```python
from build123d import *

# Parameters (mm, degrees)
SKETCH1_W           = 25
SKETCH1_H           = 15
BOSS_EXTRUDE1_DEPTH = 5
SKETCH2_R           = 1
SKETCH2_R_2         = 0.75
BOSS_EXTRUDE2_DEPTH = 5
SKETCH3_R           = 0.75
BOSS_EXTRUDE3_DEPTH = 5


with BuildPart() as part:
    # Sketch1 → Boss-Extrude1 (new body)
    with BuildSketch(Plane(origin=(0, 0, 0), x_dir=(1, 0, 0), z_dir=(0, 1, 0))):
        with Locations((12.5, 7.5)):
            Rectangle(SKETCH1_W, SKETCH1_H)
    extrude(amount=BOSS_EXTRUDE1_DEPTH)

    # Sketch2 → Boss-Extrude2 (add)
    with BuildSketch(Plane(origin=(25, 0, 0), x_dir=(0, 0, -1), z_dir=(1, 0, 0))):
        with Locations(Location((11.5, 2.5, 0), (0, 0, 180))):
            Circle(SKETCH2_R)
        with Locations(Location((6, 2.5, 0), (0, 0, 180))):
            Circle(SKETCH2_R_2)
        with Locations(Location((9, 2.5, 0), (0, 0, 180))):
            Circle(SKETCH2_R_2)
        with Locations(Location((3.5, 2.5, 0), (0, 0, 180))):
            Circle(SKETCH2_R)
    extrude(amount=BOSS_EXTRUDE2_DEPTH)

    # Sketch3 → Boss-Extrude3 (add)
    with BuildSketch(Plane.ZY):
        with Locations(Location((-9.5, 2.5, 0), (0, 0, 180))):
            Circle(SKETCH3_R)
        with Locations(Location((-7.5, 2.5, 0), (0, 0, 180))):
            Circle(SKETCH3_R)
        with Locations(Location((-5.5, 2.5, 0), (0, 0, 180))):
            Circle(SKETCH3_R)
    extrude(amount=BOSS_EXTRUDE3_DEPTH)


solid = part.part
```
Model file for the job. Use its own axes, mm. A direction names the side the tool comes from. Round coordinates to 2 decimals unless told otherwise and drop trailing zeros. Write each loop counter-clockwise with the first axis right and the second up, starting at its lowest first coordinate (ties: lowest second). Pieces come first, ordered by that corner, then holes. Notation, with made-up numbers: M -20.5,63 L 4.5,63 A14 ccw 4.5,67 Z; hole C 76.25,62.5 d7. An arc over 180 degrees is marked long. Put each result on its own line as item: value.
Item 1: Cut at D-D (x = -3). List the corners of the cut face in (y, z), and give its area (3 significant figures).
Responses:
outline: C 2.5,-9.5 d1.5; C 2.5,-7.5 d1.5; C 2.5,-5.5 d1.5
area: 5.30 mm²
Item 2: Cut at A-A (x = 27). List the corners of the cut face in (y, z), and give its area (3 significant figures).
Responses:
outline: C 2.5,-11.5 d2; C 2.5,-3.5 d2; C 2.5,-9 d1.5; C 2.5,-6 d1.5
area: 9.82 mm²
Item 3: Tool access for faces 5 (the flat face through (0, 1, -7)), 6 (the cylindrical face through (27.46, 2.47, -9.75)), 7 (the flat face through (30, 2, -6)): list every direction of +Z, -Z, +X, -X, +Y, -Y with a clear straight run to the whole face (end or side of a thin tool).
Responses:
face 5: -X
face 6: +X
face 7: +Z, -Z, +X, +Y, -Y
Item 4: Probe L1, parallel to Z at x = -3, y = 2; L2, parallel to Z at x = 27, y = 3.05; L3, parallel to X at y = 0.9, z = -10. List the from-to ranges inside material, lowest first. Write a range as from..to.
Responses:
L1: -10.06..-8.94, -8.06..-6.94, -6.06..-4.94
L2: -12.34..-10.66, -9.51..-8.49, -6.51..-5.49, -4.34..-2.66
L3: 0..25
Item 5: Mould opens along Z. For faces 1 (the flat face through (-5, 2.5, -7.5)), 2 (the cylindrical face through (-2.46, 2.47, -6.75)), 3 (the flat face through (12, 2, -15)), 4 (the cylindrical face through (27.5, 3.1, -12.3)) say: +Z half, -Z half, draft (parallel to the pull), parting line (faces both ways), or undercut.
Responses:
face 1: draft
face 2: undercut
face 3: -Z half
face 4: undercut
Item 6: Cut at C-C (z = -11.5). List the corners of the cut face in (x, y), and give its area (3 significant figures).
Responses:
outline: M 0,0 L 25,0 L 25,1.5 L 30,1.5 L 30,3.5 L 25,3.5 L 25,5 L 0,5 Z
area: 135 mm²
